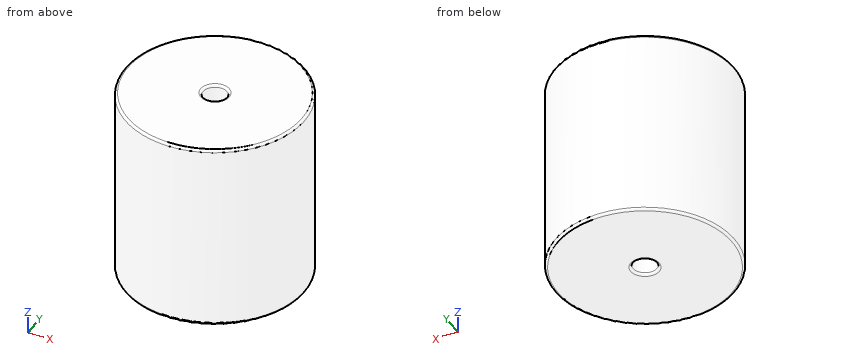
Solid Edge part; units mm, degrees
sketch "Sketch1" plane through (0, 0, 0) normal (0, 0, 1) x (1, 0, 0)
  circle A0 centre (0, 0) radius 37.5
extrude "ExtrudedProtrusion_1" add sketch "Sketch1" along normal mid plane 80
fillet "Round_1" radius 1 2 edges at (-37.5, 0, 40) (-37.5, 0, -40)
hole "Hole_1" at (0, 0, 40) direction (0, 0, -1) diameter 10 end up to next
fillet "Round_2" radius 1 2 edges at (-5, 0, 40) (5, 0, -40)
properties material "Acrylic, high impact grade"
Work out the finished part from the listing and answer in its coordinate system (mm). Round coordinates to 2 decimals unless told otherwise and drop trailing zeros. Write each loop counter-clockwise with the first axis right and the second up, starting at its lowest first coordinate (ties: lowest second). Pieces come first, ordered by that corner, then holes. Notation, with made-up numbers: M 2.25,52 L 9.25,52 A29 cw 9.25,79 Z; hole C 83,52.5 d2. An arc over 180 degrees is marked long. Use a Markdown table: item, result.
1) Consider line 1 (Y direction, x = 0, z = 21); line 2 (Y direction, x = 28, z = -3); line 3 (Y direction, x = -20.5, z = 15.5). Determine where each line is inside the solid, lowest interval first. Write a range as [from, to].
Taken from the geometry:
| item | result |
|---|---|
| line 1 | y = [-37.5, -5], [5, 37.5] |
| line 2 | y = [-24.94, 24.94] |
| line 3 | y = [-31.4, 31.4] |
2) The part is cut by section A-A on y = 0. Give the vertices of the cut face in (x, z), plus the area to 3 significant figures.
Taken from the geometry:
| item | result |
|---|---|
| outline | M -37.5,-39 A1 ccw -36.5,-40 L -6,-40 A1 ccw -5,-39 L -5,39 A1 ccw -6,40 L -36.5,40 A1 ccw -37.5,39 Z; M 5,-39 A1 ccw 6,-40 L 36.5,-40 A1 ccw 37.5,-39 L 37.5,39 A1 ccw 36.5,40 L 6,40 A1 ccw 5,39 Z |
| area | 5,200 mm2 |
3) The part is cut by section C-C on z = -7.5. Give the vertices of the cut face in (x, y), plus the area to 3 significant figures.
Taken from the geometry:
| item | result |
|---|---|
| outline | C 0,0 d75; hole C 0,0 d10 |
| area | 4,340 mm2 |
4) Flat-ended cylindrical pins translate along their axes: pin 1 (5 mm diameter, centred on y = -21, z = -12, fed in from -X); pin 2 (1.5 mm diameter, centred on x = -23.5, z = 21, fed in from -Y); pin 3 (5 mm diameter, centred on y = -20, z = -15.5, fed in from +X). Find the tip coordinate at first contact, or state that the pin passes through.
Taken from the geometry:
| item | result |
|---|---|
| pin 1 | stops at x = -32.62 |
| pin 2 | stops at y = -29.81 |
| pin 3 | stops at x = 33.17 |
